Work out the finished part from the listing and answer in its coordinate system (mm). Coordinates: 2 decimals unless noted, no trailing zeros. Loops run counter-clockwise (first coordinate to the right, second up) from the corner with the lowest first, then second, coordinate; pieces in that order, holes last. Notation, with made-up numbers: (79.5, 6) -> (92.5, 6) arc R27 ccw to (92.5, 45) -> close; hole circle Ø2 at (19, -32). An arc over 180 degrees is marked (long way). One line per question, with ' | ' between items.
```python
from build123d import *

# Parameters (mm, degrees)
BOSS_EXTRUDE1_DEPTH     = 1.5875
FILLET1_R               = 1.27
SKETCH2_R               = 0.635
CUT_EXTRUDE1_DEPTH      = 1
CUT_EXTRUDE1_DEPTH_BACK = 2.5875


with BuildPart() as part:
    # Sketch1 → Boss-Extrude1 (new body)
    with BuildSketch(Plane(origin=(0, 0, 0), x_dir=(1, 0, 0), z_dir=(0, 1, 0))):
        with BuildLine():
            Line((-66.675, 3.175), (-66.675, 55.209357386))
            Line((-66.675, 55.209357386), (-58.801, 55.209357386))
            Line((-58.801, 55.209357386), (-58.801, 36.83))
            Line((-58.801, 36.83), (-24.765, 36.83))
            Line((-24.765, 36.83), (-24.765, 3.175))
            Line((-24.765, 3.175), (24.765, 3.175))
            Line((24.765, 3.175), (24.765, 62.865))
            Line((24.765, 62.865), (62.23, 62.865))
            ThreePointArc((62.23, 62.865), (63.128025612, 62.493025612), (63.5, 61.595))
            ThreePointArc((63.5, 61.595), (63.871974388, 60.696974388), (64.77, 60.325))
            Line((64.77, 60.325), (66.675, 60.325))
            Line((66.675, 60.325), (66.675, 3.175))
            ThreePointArc((66.675, 3.175), (65.74506403, 0.92993597), (63.5, 0))
            Line((63.5, 0), (-63.5, 0))
            ThreePointArc((-63.5, 0), (-65.74506403, 0.92993597), (-66.675, 3.175))
        make_face()
    extrude(amount=BOSS_EXTRUDE1_DEPTH)

    # Fillet1
    fillet1_edges = [part.edges().sort_by_distance(p)[0] for p in [
        (-58.801, 0.79375, -55.209357386),
        (-58.801, 0.79375, -36.83),
        (-24.765, 0.79375, -36.83),
    ]]
    fillet(fillet1_edges, radius=FILLET1_R)

    # Sketch2 → Cut-Extrude1 (cut, two sides)
    with BuildSketch(Plane(origin=(0, 1.5875, 0), x_dir=(-1, 0, 0), z_dir=(0, 1, 0))) as cut_extrude1_sk:
        with Locations((63.074630657, -1.5875)):
            Circle(SKETCH2_R)
        with Locations((50.459704526, -1.5875)):
            Circle(SKETCH2_R)
        with Locations((37.844778394, -1.5875)):
            Circle(SKETCH2_R)
        with Locations((25.229852263, -1.5875)):
            Circle(SKETCH2_R)
        with Locations((12.614926131, -1.5875)):
            Circle(SKETCH2_R)
        with Locations((0, -1.5875)):
            Circle(SKETCH2_R)
        with Locations((-12.614926131, -1.5875)):
            Circle(SKETCH2_R)
        with Locations((-25.229852263, -1.5875)):
            Circle(SKETCH2_R)
        with Locations((-37.844778394, -1.5875)):
            Circle(SKETCH2_R)
        with Locations((-50.459704526, -1.5875)):
            Circle(SKETCH2_R)
        with Locations((-63.074630657, -1.5875)):
            Circle(SKETCH2_R)
        with Locations((63.074630657, -14.199214347)):
            Circle(SKETCH2_R)
        with Locations((63.074630657, -26.810928693)):
            Circle(SKETCH2_R)
        with Locations((63.074630657, -39.42264304)):
            Circle(SKETCH2_R)
        with Locations((63.074630657, -52.034357386)):
            Circle(SKETCH2_R)
        with Locations((-63.074630657, -15.750103912)):
            Circle(SKETCH2_R)
        with Locations((-63.074630657, -29.912707823)):
            Circle(SKETCH2_R)
        with Locations((-63.074630657, -44.075311735)):
            Circle(SKETCH2_R)
        with Locations((-62.100867444, -59.69)):
            Circle(SKETCH2_R)
        with Locations((-50.713911629, -59.69)):
            Circle(SKETCH2_R)
        with Locations((-39.326955815, -59.69)):
            Circle(SKETCH2_R)
        with Locations((-27.94, -59.69)):
            Circle(SKETCH2_R)
        with Locations((-27.94, -45.958125)):
            Circle(SKETCH2_R)
        with Locations((-27.94, -32.22625)):
            Circle(SKETCH2_R)
        with Locations((-27.94, -18.494375)):
            Circle(SKETCH2_R)
        with Locations((-27.94, -4.7625)):
            Circle(SKETCH2_R)
    extrude(amount=CUT_EXTRUDE1_DEPTH, mode=Mode.SUBTRACT)
    extrude(cut_extrude1_sk.sketch, amount=-CUT_EXTRUDE1_DEPTH_BACK, mode=Mode.SUBTRACT)


solid = part.part
```
1) Find section A-A (z = -11). Write down the section's boundary in (x, y) (1 decimal), plus the area to 3 significant figures.
Check values:
outline: (-66.7, 0) -> (-24.8, 0) -> (-24.8, 1.6) -> (-66.7, 1.6) -> close; (24.8, 0) -> (66.7, 0) -> (66.7, 1.6) -> (24.8, 1.6) -> close | area: 133 mm^2
2) Find section C-C (y = 0.8). State how many separate pieces and enclosed holes the cut face has, plus the area to 3 significant figures.
Check values:
separate pieces: 1 | enclosed holes: 26 | area: 4,430 mm^2
3) Find the intervals of material crossed by line 1 along X through (y, z) = (1.4, -30) (3 decimals); line 2 along X through (y, z) = (0.15, -25.5) (3 decimals); line 3 along X through (y, z) = (1.15, -50) (3 decimals), in increasing order.
Check values:
line 1: x = -66.675 to -24.765, 24.765 to 62.446, 63.704 to 66.675 | line 2: x = -66.675 to -24.765, 24.765 to 66.675 | line 3: x = -66.675 to -58.801, 24.765 to 66.675
4) Find section B-B (x = -5.5). Write down the section's boundary in (y, z) (1 decimal), plus the area to 3 significant figures.
Check values:
outline: (0, -3.2) -> (1.6, -3.2) -> (1.6, 0) -> (0, 0) -> close | area: 5.04 mm^2
